Design review of the part shown in the three views and the two pictorial views. Dimensions are in mm from the part's minimum x, y and z. A direction names the side the tool comes from. Round coordinates to 2 decimals unless told otherwise and drop trailing zeros. Loops run counter-clockwise (first coordinate to the right, second up) from the corner with the lowest first, then second, coordinate; pieces in that order, holes last.
1. Consider section C-C on z = 11. State how many separate pieces and enclosed holes the cut face has, then the cut area to 3 significant figures.
2. Clearance check with a flat-ended pin moving along its axis: pin 1 Ø8 at (x, y) = (26.5, 45.5) entering from +Z. State where the tip first meets the part, or that it passes through.
3. Consider section D-D on x = 37. State the section outline as (y, z) points.
4. Draft analysis for pull direction X (two halves, no side actions). For the marked faces 3, 4, 5 and 6, state which applies: released by +X, released by -X, zero draft, split by the parting line, or undercut.
5. Consider section B-B on y = 39.5. State the section outline as (x, z) points.
6. Tool access review of the marked faces 1 and 2: name each direction out of +Z, -Z, +X, -X, +Y, -Y from which nothing blocks a thin tool from reaching the whole face with its end or side.
7. Consider section A-A on x = 12. State the section outline as (y, z) points.
8. To check wall thickness, follow line 1 along Y through (x, z) = (36, 14); line 2 along X through (y, z) = (74.5, 23.5); line 3 along Y through (x, z) = (34.5, 19.5). State the ranges of each line that lie inside material, in increasing order.
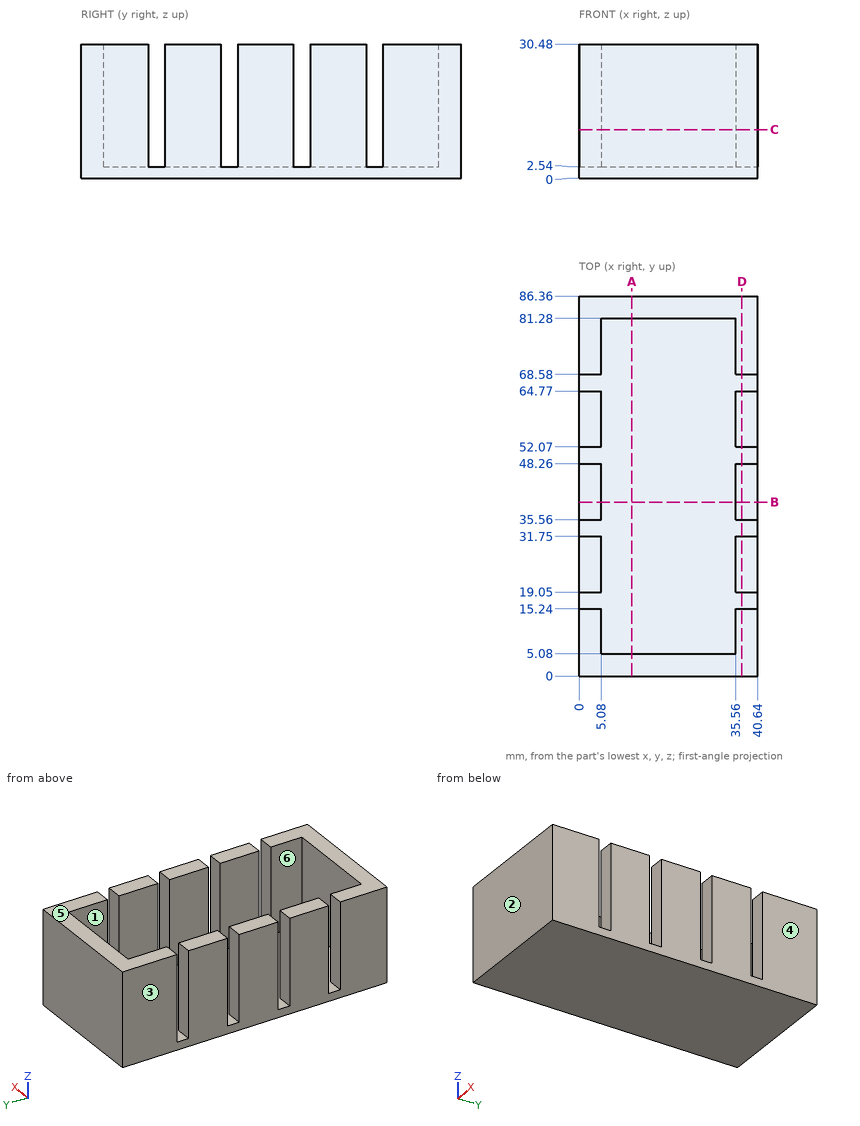
Resolved:
1. separate pieces: 8
1. enclosed holes: 0
1. area: 1,030 mm2
2. pin 1: stops at z = 2.54
3. outline: (0, 0) - (86.36, 0) - (86.36, 30.48) - (68.58, 30.48) - (68.58, 2.54) - (64.77, 2.54) - (64.77, 30.48) - (52.07, 30.48) - (52.07, 2.54) - (48.26, 2.54) - (48.26, 30.48) - (35.56, 30.48) - (35.56, 2.54) - (31.75, 2.54) - (31.75, 30.48) - (19.05, 30.48) - (19.05, 2.54) - (15.24, 2.54) - (15.24, 30.48) - (0, 30.48) - close
4. face 3: released by -X
4. face 4: released by +X
4. face 5: zero draft
4. face 6: undercut
5. outline: (0, 0) - (40.64, 0) - (40.64, 30.48) - (35.56, 30.48) - (35.56, 2.54) - (5.08, 2.54) - (5.08, 30.48) - (0, 30.48) - close
6. face 1: +Z
6. face 2: +Z, -Z, +X, -X, -Y
7. outline: (0, 0) - (86.36, 0) - (86.36, 30.48) - (81.28, 30.48) - (81.28, 2.54) - (5.08, 2.54) - (5.08, 30.48) - (0, 30.48) - close
8. line 1: y = 0 to 15.24, 19.05 to 31.75, 35.56 to 48.26, 52.07 to 64.77, 68.58 to 86.36
8. line 2: x = 0 to 5.08, 35.56 to 40.64
8. line 3: y = 0 to 5.08, 81.28 to 86.36
